Can you work these out from the model? Positions are in its coordinate system, mm. A direction names the side the tool comes from. Round coordinates to 2 decimals unless told otherwise and drop trailing zeros. Order: outer loops, then holes, each group sorted by start corner. A loop starts at its lowest first (then second) coordinate and runs counter-clockwise, first axis right, second up.
Q1. If we section it at C-C (x = -105.5): Please give me the cut outline in (y, z).
Q2. We'd pull the mould along Z, two halves only. Please class faces 1 (the face through (-106.974, -14.048, -8.387)), 2 (the face through (-107, -23, -22)), 3 (the face through (-106, -24, -9.735)): pulls with the +Z half, pulls with the -Z half, needs draft (parallel to the pull), parting line crosses it, or undercut.
Q3. If we section it at B-B (x = -108): Please give me the cut outline in (y, z), plus the area to 3 significant figures.
Q4. If I drill on line 1 (Y direction, x = -105.5, z = -8.3); line 2 (Z direction, x = -107.5, y = -26.75); line 3 (X direction, y = -15.4, z = -20.6), over which ranges is the centre line in solid material (lowest first)?
Q5. If we section it at D-D (z = -20): Please give me the cut outline in (x, y).
Q6. For faces 4 (the face through (-106, -29, -13.235)), 5 (the face through (-107, -9, -15)), which set-ups out of +Z, -Z, +X, -X, +Y, -Y let a thin tool reach every point of the face, with its end or its side?
Q7. If we section it at A-A (y = -15.4): Please give me the cut outline in (x, z), plus the area to 3 significant figures.
from build123d import *

# Parameters (mm, degrees)
CYLINDER011_R     = 2
CYLINDER011_DEPTH = 50
PAD002_DEPTH      = 30
BOX007_W          = 10
BOX007_H          = 28
BOX007_DEPTH      = 15


with BuildPart() as cylinder011:
    # Cylinder011 → Cylinder011 (new body)
    with BuildSketch(Plane(origin=(-105.5, -15.4, -37), x_dir=(1, 0, 0), z_dir=(0, 0, 1))):
        Circle(CYLINDER011_R)
    extrude(amount=CYLINDER011_DEPTH)


with BuildPart() as fusion001006:
    # Sketch002 → Pad002 (new body)
    with BuildSketch(Plane.YZ):
        Polygon((-36.805373, -9.734821), (-11.122054, -9.734821), (-11.122054, -16.734821), (-20.919355, -16.734821), (-20.919355, -13.234821), (-36.805373, -13.234821), align=None)
    extrude(amount=PAD002_DEPTH)


with BuildPart() as fusion001006_1:
    # Body002 placement: moved
    add(fusion001006.part.moved(Location((-110, 0, 0))))

    # Fusion001006: union Cylinder011
    add(cylinder011.part)


with BuildPart() as cut010:
    # Box007 → Box007 (new body)
    with BuildSketch(Plane(origin=(-112, -37, -22), x_dir=(1, 0, 0), z_dir=(0, 0, 1))):
        with Locations((5, 14)):
            Rectangle(BOX007_W, BOX007_H)
    extrude(amount=BOX007_DEPTH)

    # Cut010: cut Fusion001006
    add(fusion001006_1.part, mode=Mode.SUBTRACT)


solid = cut010.part
Solution:
1. outline: (-37, -22) - (-17.4, -22) - (-17.4, -16.73) - (-20.92, -16.73) - (-20.92, -13.23) - (-36.81, -13.23) - (-36.81, -9.73) - (-17.4, -9.73) - (-17.4, -7) - (-37, -7) - close; (-13.4, -22) - (-9, -22) - (-9, -7) - (-13.4, -7) - (-13.4, -9.73) - (-11.12, -9.73) - (-11.12, -16.73) - (-13.4, -16.73) - close
2. face 1: needs draft
2. face 2: pulls with the -Z half
2. face 3: undercut
3. outline: (-37, -22) - (-9, -22) - (-9, -7) - (-37, -7) - close; hole (-36.81, -13.23) - (-20.92, -13.23) - (-20.92, -16.73) - (-11.12, -16.73) - (-11.12, -9.73) - (-36.81, -9.73) - close
3. area: 296 mm2
4. line 1: y = -37 to -17.4, -13.4 to -9
4. line 2: z = -22 to -13.23, -9.73 to -7
4. line 3: x = -112 to -107.5, -103.5 to -102
5. outline: (-112, -37) - (-102, -37) - (-102, -9) - (-112, -9) - close; hole circle Ø4 at (-105.5, -15.4)
6. face 4: +X
6. face 5: +Z, -Z, +X, -X, +Y
7. outline: (-112, -22) - (-107.5, -22) - (-107.5, -16.73) - (-110, -16.73) - (-110, -9.73) - (-107.5, -9.73) - (-107.5, -7) - (-112, -7) - close; (-103.5, -22) - (-102, -22) - (-102, -16.73) - (-103.5, -16.73) - close; (-103.5, -9.73) - (-102, -9.73) - (-102, -7) - (-103.5, -7) - close
7. area: 62.0 mm2
